The listing builds one solid part. Answer for the finished solid, in the listing's coordinates (mm). A direction names the side the tool comes from. Give positions to 0.01 mm unless a question says otherwise; leave off trailing zeros. Order: outer loops, then holes, each group sorted by start corner. A loop starts at its lowest first (then second) coordinate and runs counter-clockwise, first axis right, second up. Notation, with made-up numbers: M 15,-18 L 22,-18 A20 ccw 22,13 Z; hole C 16.5,35.5 d7. An arc over 180 degrees is marked long. Answer as a JSON object with one key per item and string values. Group by question number.
```python
from build123d import *

# Parameters (mm, degrees)
SKETCH1_R           = 1.6
SKETCH1_W           = 20.6
SKETCH1_H           = 2.4
SKETCH1_W_2         = 36
SKETCH1_H_2         = 10
SKETCH1_W_3         = 15.54
SKETCH1_W_4         = 25.66
SKETCH1_W_5         = 20.65
SKETCH1_W_6         = 9.5
SKETCH1_H_3         = 12.3
SKETCH1_W_7         = 11
SKETCH1_H_4         = 9
BOSS_EXTRUDE1_DEPTH = 1.6
SKETCH1_3_W         = 6.7
SKETCH1_3_H         = 12.3
SKETCH1_3_W_2       = 9.5
BOSS_EXTRUDE2_DEPTH = 10.7
SKETCH1_4_W         = 11
SKETCH1_4_H         = 9
SKETCH1_4_W_2       = 2.6
BOSS_EXTRUDE3_DEPTH = 11
SKETCH1_5_W         = 36
SKETCH1_5_H         = 10
BOSS_EXTRUDE4_DEPTH = 8
SKETCH1_6_W         = 25.66
SKETCH1_6_H         = 2.4
SKETCH1_6_W_2       = 20.65
SKETCH1_6_W_3       = 15.54
SKETCH1_6_W_4       = 20.6
BOSS_EXTRUDE5_DEPTH = 8.5


with BuildPart() as part:
    # Sketch1 → Boss-Extrude1 (new body)
    # profile 1 of 8: a face of its own
    with BuildSketch(Plane(origin=(0, 0, 0), x_dir=(1, 0, 0), z_dir=(0, 1, 0))):
        Polygon((68.7, 38.5), (66.2, 41), (66.2, 53.2), (0, 53.2), (0, 44.2), (9.5, 44.2), (9.5, 31.9), (0, 31.9), (0, 12.3), (11, 12.3), (11, 3.3), (0, 3.3), (0, 0), (66.2, 0), (66.2, 3), (68.7, 5.5), align=None)
        with Locations(Location((13.5, 2.5, 0), (0, 0, 270))):
            Circle(SKETCH1_R, mode=Mode.SUBTRACT)
        with Locations((36.86, 2.8)):
            Rectangle(SKETCH1_W, SKETCH1_H, mode=Mode.SUBTRACT)
        with Locations((45.5, 12.617620005)):
            Rectangle(SKETCH1_W_2, SKETCH1_H_2, mode=Mode.SUBTRACT)
        with Locations((57.03, 2.8)):
            Rectangle(SKETCH1_W_3, SKETCH1_H, mode=Mode.SUBTRACT)
        with Locations(Location((66.2, 8, 0), (0, 0, 270))):
            Circle(SKETCH1_R, mode=Mode.SUBTRACT)
        with Locations(Location((15, 50.7, 0), (0, 0, 270))):
            Circle(SKETCH1_R, mode=Mode.SUBTRACT)
        with Locations((29.63, 50.7)):
            Rectangle(SKETCH1_W_4, SKETCH1_H, mode=Mode.SUBTRACT)
        with Locations(Location((66.2, 36, 0), (0, 0, 270))):
            Circle(SKETCH1_R, mode=Mode.SUBTRACT)
        with Locations((54.475, 50.9)):
            Rectangle(SKETCH1_W_5, SKETCH1_H, mode=Mode.SUBTRACT)
    # profile 2 of 8: a face of its own
    with BuildSketch(Plane(origin=(0, 0, 0), x_dir=(1, 0, 0), z_dir=(0, 1, 0))):
        with Locations((4.75, 38.05)):
            Rectangle(SKETCH1_W_6, SKETCH1_H_3)
    # profile 3 of 8: a face of its own
    with BuildSketch(Plane(origin=(0, 0, 0), x_dir=(1, 0, 0), z_dir=(0, 1, 0))):
        with Locations((5.5, 7.8)):
            Rectangle(SKETCH1_W_7, SKETCH1_H_4)
    # profile 4 of 8: a face of its own
    with BuildSketch(Plane(origin=(0, 0, 0), x_dir=(1, 0, 0), z_dir=(0, 1, 0))):
        with Locations((45.5, 12.617620005)):
            Rectangle(SKETCH1_W_2, SKETCH1_H_2)
    # profile 5 of 8: a face of its own
    with BuildSketch(Plane(origin=(0, 0, 0), x_dir=(1, 0, 0), z_dir=(0, 1, 0))):
        with Locations((36.86, 2.8)):
            Rectangle(SKETCH1_W, SKETCH1_H)
    # profile 6 of 8: a face of its own
    with BuildSketch(Plane(origin=(0, 0, 0), x_dir=(1, 0, 0), z_dir=(0, 1, 0))):
        with Locations((57.03, 2.8)):
            Rectangle(SKETCH1_W_3, SKETCH1_H)
    # profile 7 of 8: a face of its own
    with BuildSketch(Plane(origin=(0, 0, 0), x_dir=(1, 0, 0), z_dir=(0, 1, 0))):
        with Locations((29.63, 50.7)):
            Rectangle(SKETCH1_W_4, SKETCH1_H)
    # profile 8 of 8: a face of its own
    with BuildSketch(Plane(origin=(0, 0, 0), x_dir=(1, 0, 0), z_dir=(0, 1, 0))):
        with Locations((54.475, 50.9)):
            Rectangle(SKETCH1_W_5, SKETCH1_H)
    extrude(amount=-BOSS_EXTRUDE1_DEPTH)

    # Sketch1_3 → Boss-Extrude2 (add)
    with BuildSketch(Plane(origin=(0, 0, 0), x_dir=(1, 0, 0), z_dir=(0, 1, 0))):
        with Locations((-3.35, 38.05)):
            Rectangle(SKETCH1_3_W, SKETCH1_3_H)
        with Locations((4.75, 38.05)):
            Rectangle(SKETCH1_3_W_2, SKETCH1_3_H)
    extrude(amount=BOSS_EXTRUDE2_DEPTH)

    # Sketch1_4 → Boss-Extrude3 (add)
    with BuildSketch(Plane(origin=(0, 0, 0), x_dir=(1, 0, 0), z_dir=(0, 1, 0))):
        with Locations((5.5, 7.8)):
            Rectangle(SKETCH1_4_W, SKETCH1_4_H)
        with Locations((-1.3, 7.8)):
            Rectangle(SKETCH1_4_W_2, SKETCH1_4_H)
    extrude(amount=BOSS_EXTRUDE3_DEPTH)

    # Sketch1_5 → Boss-Extrude4 (add)
    with BuildSketch(Plane(origin=(0, 0, 0), x_dir=(1, 0, 0), z_dir=(0, 1, 0))):
        with Locations((45.5, 12.617620005)):
            Rectangle(SKETCH1_5_W, SKETCH1_5_H)
    extrude(amount=BOSS_EXTRUDE4_DEPTH)

    # Sketch1_6 → Boss-Extrude5 (add)
    with BuildSketch(Plane(origin=(0, 0, 0), x_dir=(1, 0, 0), z_dir=(0, 1, 0))):
        with Locations((29.63, 50.7)):
            Rectangle(SKETCH1_6_W, SKETCH1_6_H)
        with Locations((54.475, 50.9)):
            Rectangle(SKETCH1_6_W_2, SKETCH1_6_H)
        with Locations((57.03, 2.8)):
            Rectangle(SKETCH1_6_W_3, SKETCH1_6_H)
        with Locations((36.86, 2.8)):
            Rectangle(SKETCH1_6_W_4, SKETCH1_6_H)
    extrude(amount=BOSS_EXTRUDE5_DEPTH)


solid = part.part
```
Item 1: Section B-B (y = 5) is taken. Determine the outline of the cut face in (x, z), and give its area (3 significant figures).
Item 2: Consider probe 1 along Z at (x, y) = (45.5, 7.25); probe 2 along Z at (x, y) = (36, 3.25); probe 3 along X at (y, z) = (-0.8, -50.7). Determine where each line is inside the solid, lowest interval first. Write a range as from..to.
Item 3: Section A-A (z = -50.7) is taken. Determine the outline of the cut face in (x, y), and give its area (3 significant figures).
Item 4: Flat-ended cylindrical pins translate along their axes: P1, Ø1.3, axis at x = -2, z = -6.5, coming from the -Y side; P2, Ø5, axis at y = 3.5, z = -8.5, coming from the -X side; P3, Ø3.5, axis at x = 0, z = -40, coming from the +Y side. Find the tip coordinate at first contact, or state that the pin passes through.
Item 5: A tool of negligible diameter and unlimited length cuts with its end or side. For faces 4 (the flat face through (1, 5, -31.9)), 5 (the flat face through (-3, 0, -38)), 6 (the flat face through (57, 4, -1.6)), 7 (the flat face through (26.56, 4, -3)), from which of +Z, -Z, +X, -X, +Y, -Y can it reach the whole face along a straight path? Write none if from no direction.
Item 6: Determine the mould class of faces 1 (the flat face through (47.16, 4, -3)), 2 (the flat face through (29, 4, -51.9)), 3 (the flat face through (-2.6, 5, -8)) for opening direction X: released by +X, released by -X, zero draft, split by the parting line, or undercut.
Item 7: Section C-C (x = 8) is taken. Determine the outline of the cut face in (y, z).
Item 8: Section D-D (z = -36) is taken. Determine the outline of the cut face in (x, y), and give its area (3 significant figures).
Values found:
{
 "1": {"outline": "M -6.7,-44.2 L 9.5,-44.2 L 9.5,-31.9 L -6.7,-31.9 Z; M -2.6,-12.3 L 11,-12.3 L 11,-3.3 L -2.6,-3.3 Z; M 16.8,-51.9 L 42.46,-51.9 L 42.46,-49.5 L 16.8,-49.5 Z; M 26.56,-4 L 47.16,-4 L 47.16,-1.6 L 26.56,-1.6 Z; M 27.5,-17.62 L 63.5,-17.62 L 63.5,-7.62 L 27.5,-7.62 Z; M 44.15,-52.1 L 64.8,-52.1 L 64.8,-49.7 L 44.15,-49.7 Z; M 49.26,-4 L 64.8,-4 L 64.8,-1.6 L 49.26,-1.6 Z", "area": "880 mm^2"},
 "2": {"probe 1": "z = -52.1..-49.7, -17.62..-7.62, -4..-1.6", "probe 2": "z = -51.9..-49.5, -17.62..-7.62, -4..-1.6", "probe 3": "x = 0..13.4, 16.6..66.2"},
 "3": {"outline": "M 0,-1.6 L 13.4,-1.6 L 13.4,0 L 0,0 Z; M 16.6,-1.6 L 66.2,-1.6 L 66.2,0 L 64.8,0 L 64.8,8.5 L 44.15,8.5 L 44.15,0 L 42.46,0 L 42.46,8.5 L 16.8,8.5 L 16.8,0 L 16.6,0 Z", "area": "494 mm^2"},
 "4": {"P1": "stops at y = 0", "P2": "stops at x = -2.6", "P3": "stops at y = 10.7"},
 "5": {"face 4": "+X, -X, +Y", "face 5": "+Z, -Z, -X, -Y", "face 6": "+Z, +X, -X, +Y", "face 7": "+Z, +Y"},
 "6": {"face 1": "undercut", "face 2": "zero draft", "face 3": "released by -X"},
 "7": {"outline": "M -1.6,-53.2 L 0,-53.2 L 0,-44.2 L 10.7,-44.2 L 10.7,-31.9 L 0,-31.9 L 0,-12.3 L 11,-12.3 L 11,-3.3 L 0,-3.3 L 0,0 L -1.6,0 Z"},
 "8": {"outline": "M -6.7,0 L 0,0 L 0,-1.6 L 64.6,-1.6 L 64.6,0 L 9.5,0 L 9.5,10.7 L -6.7,10.7 Z; M 67.8,-1.6 L 68.7,-1.6 L 68.7,0 L 67.8,0 Z", "area": "278 mm^2"}
}
